from build123d import *
from build123d.topology import SkipClean

# Parameters (mm, degrees)
SKETCH1_R           = 2.85
SKETCH1_R_2         = 1
BOSS_EXTRUDE1_DEPTH = 7.85
CUT_SWEEP3_PITCH    = 1.5


with BuildPart() as part:
    # Sketch1 → Boss-Extrude1 (new body)
    with BuildSketch(Plane(origin=(0, 0, 0), x_dir=(0, 0, -1), z_dir=(1, 0, 0))):
        Circle(SKETCH1_R)
        Circle(SKETCH1_R_2, mode=Mode.SUBTRACT)
    extrude(amount=BOSS_EXTRUDE1_DEPTH)

    # Cut-Sweep3: the profile of Sketch3 screwed along a right-hand helix of 6.5 turns, 8 arcs to a turn; built about Z, then put on its axis
    with SkipClean():  # the faces are left unmerged after this step: merging them gives an invalid solid
        cut_sweep3_z = Axis((0, 0, 0), (0, 0, 1))
        cut_sweep3_corners = [(2.85, 0, 0), (1.85, 0, -0.75), (2.85, 0, -1.5), (3.101496865, 0, -1.5), (3.101496865, 0, 0)]
        with BuildLine(mode=Mode.PRIVATE) as cut_sweep3_profile:
            Line(cut_sweep3_corners[0], cut_sweep3_corners[1])
            Line(cut_sweep3_corners[1], cut_sweep3_corners[2])
            Line(cut_sweep3_corners[2], cut_sweep3_corners[3])
            Line(cut_sweep3_corners[3], cut_sweep3_corners[4])
            Line(cut_sweep3_corners[4], cut_sweep3_corners[0])
        cut_sweep3_cap = Face(cut_sweep3_profile.wire())
        cut_sweep3_turn_angles = [0, 22.5, 45, 67.5, 90, 112.5, 135, 157.5, 180, 202.5, 225, 247.5, 270, 292.5, 315, 337.5, 360]
        cut_sweep3_turn_weights = [1, 0.9238795325112867, 1, 0.9238795325112867, 1, 0.9238795325112867, 1, 0.9238795325112867, 1, 0.9238795325112867, 1, 0.9238795325112867, 1, 0.9238795325112867, 1, 0.9238795325112867, 1]
        cut_sweep3_turn_rails = [Edge.make_bspline([Vector(p[0], p[1], 0).rotate(cut_sweep3_z, cut_sweep3_turn_angles[k]) / cut_sweep3_turn_weights[k] + Vector(0, 0, p[2] + CUT_SWEEP3_PITCH * cut_sweep3_turn_angles[k] / 360) for k in range(17)], [0, 0, 0, 1, 1, 2, 2, 3, 3, 4, 4, 5, 5, 6, 6, 7, 7, 8, 8, 8], 2, cut_sweep3_turn_weights) for p in cut_sweep3_corners]
        cut_sweep3_turn_sides = [Face.make_surface_from_curves(cut_sweep3_turn_rails[p[0]], cut_sweep3_turn_rails[p[1]]) for p in [(0, 1), (1, 2), (2, 3), (3, 4), (4, 0)]]
        cut_sweep3_turn = Solid(Shell([*cut_sweep3_turn_sides, cut_sweep3_cap, cut_sweep3_cap.rotate(cut_sweep3_z, 360).moved(Location((0, 0, CUT_SWEEP3_PITCH * 360 / 360)))]))
        cut_sweep3_last_angles = [2160, 2182.5, 2205, 2227.5, 2250, 2272.5, 2295, 2317.5, 2340]
        cut_sweep3_last_weights = [1, 0.9238795325112867, 1, 0.9238795325112867, 1, 0.9238795325112867, 1, 0.9238795325112442, 1]
        cut_sweep3_last_rails = [Edge.make_bspline([Vector(p[0], p[1], 0).rotate(cut_sweep3_z, cut_sweep3_last_angles[k]) / cut_sweep3_last_weights[k] + Vector(0, 0, p[2] + CUT_SWEEP3_PITCH * cut_sweep3_last_angles[k] / 360) for k in range(9)], [0, 0, 0, 1, 1, 2, 2, 3, 3, 4, 4, 4], 2, cut_sweep3_last_weights) for p in cut_sweep3_corners]
        cut_sweep3_last_sides = [Face.make_surface_from_curves(cut_sweep3_last_rails[p[0]], cut_sweep3_last_rails[p[1]]) for p in [(0, 1), (1, 2), (2, 3), (3, 4), (4, 0)]]
        cut_sweep3_last = Solid(Shell([*cut_sweep3_last_sides, cut_sweep3_cap.rotate(cut_sweep3_z, 2160).moved(Location((0, 0, CUT_SWEEP3_PITCH * 2160 / 360))), cut_sweep3_cap.rotate(cut_sweep3_z, 2340).moved(Location((0, 0, CUT_SWEEP3_PITCH * 2340 / 360)))]))
        cut_sweep3_each = [*[cut_sweep3_turn.moved(Location((0, 0, CUT_SWEEP3_PITCH * i))) for i in range(6)], cut_sweep3_last]
        add(Plane(origin=(7.85, 0, 0), x_dir=(0, 1, 0), z_dir=(-1, 0, 0)) * Compound([cut_sweep3_each[i] for i in range(0, 7, 2)]), mode=Mode.SUBTRACT)
        add(Plane(origin=(7.85, 0, 0), x_dir=(0, 1, 0), z_dir=(-1, 0, 0)) * Compound([cut_sweep3_each[i] for i in range(1, 7, 2)]), mode=Mode.SUBTRACT)


solid = part.part
Source: CAD feature listing. Evaluate the final solid. Frame: model axes, mm. Round coordinates to 2 decimals unless told otherwise and drop trailing zeros. Write item = value, one per line. Start each with the question number.
(1) Ray query, line 1 along X through (y, z) = (2.1, -0.95); line 2 along X through (y, z) = (2.05, -1.6); line 3 along Y through (x, z) = (0.5, 0.4). Return the intervals inside material, ascending. Write a range as from..to.
(2) Pin query (flat end, axial travel): pin 1 (1.5 mm diameter, centred on x = 2, z = 1.5, fed in from -Y); pin 2 (2 mm diameter, centred on x = 2, z = 1, fed in from +Y); pin 3 (1 mm diameter, centred on x = 5.5, y = 1, fed in from -Z). Return the tip coordinate at first contact, or that it passes through.
(3) Pull-direction query (Y, two-part tool) for faces 1 (the face through (4, -1, 0)), 2 (the face through (7.85, 1, 1)); classes: +Y half, -Y half, draft (parallel to the pull), parting line (faces both ways), or undercut.
Conclusion:
q1.line_1 = 0..0.66, 1.34..2.16, 2.84..3.66, 4.34..5.16, 5.84..6.66, 7.34..7.85
q1.line_2 = 0..0.38, 1.5..1.88, 3..3.38, 4.5..4.88, 6..6.38, 7.5..7.85
q1.line_3 = -2.07..-0.92, 0.92..2.67
q2.pin_1 = -2.68
q2.pin_2 = 2.85
q2.pin_3 = -2.62
q3.face_1 = undercut
q3.face_2 = draft
